The listing builds one solid part. Answer for the finished solid, in the listing's coordinates (mm). Face numbers are marked on the shaded views. A direction names the side the tool comes from. Round coordinates to 2 decimals unless told otherwise and drop trailing zeros. Write each loop counter-clockwise with the first axis right and the second up, starting at its lowest first coordinate (ties: lowest second). Pieces come first, ordered by that corner, then holes.
(1) A cutting plane is placed at A-A, the plane z = 0. Give the vertices of the cut face in (x, y) (3 decimals).
(2) A cutting plane is placed at D-D, the plane x = 34.5. Give the vertices of the cut face in (y, z) (3 decimals), and give its area (3 significant figures).
(3) Each of these flat-tipped pins is pushed along its axis until it touches: pin 1 Ø3 at (x, z) = (59.5, -6) entering from +Y; pin 2 Ø3 at (x, y) = (44, -3.5) entering from +Z; pin 3 Ø8 at (x, z) = (63, -6) entering from -Y; pin 4 Ø10 at (x, y) = (79, -0.5) entering from -Z (3 decimals). Where does it stop, or does it pass through?
(4) For the marked faces 1 and 2, determine the directions among +Z, -Z, +X, -X, +Y, -Y from which every point of the face is accessible in a straight line to the end or side of a thin tool.
(5) Find the intervals of material crossed by probe 1 along X at (y, z) = (3, 5.5); probe 2 along Z at (x, y) = (57, 1.75); probe 3 along Z at (x, y) = (98, -8), in increasing order.
(6) A cutting plane is placed at C-C, the plane x = 103.5. Give the vertices of the cut face in (y, z), and give its area (3 significant figures).
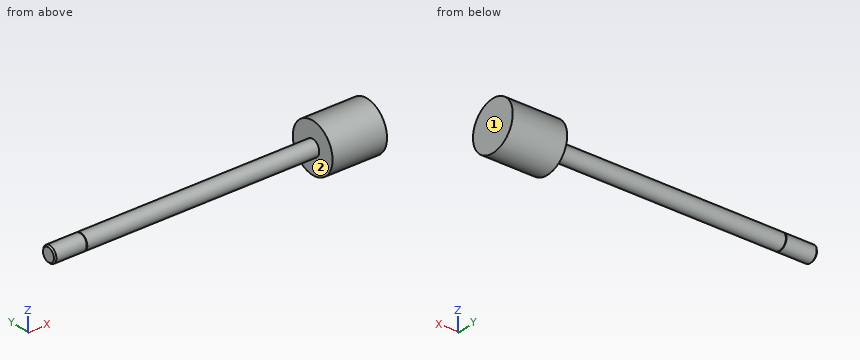
from build123d import *

# Parameters (mm, degrees)
SKETCH3_W = 0.254
SKETCH3_H = 0.508


with BuildPart() as part:
    # Sketch1 → Revolve1 (revolve)
    with BuildSketch(Plane.XY):
        Polygon((0, 0), (0, 3.175), (91.2876, 3.175), (91.2876, 9.62025), (112.7252, 9.62025), (112.7252, 0), align=None)
    revolve(axis=Axis((112.7252, 0, 0), (-1, 0, 0)))

    # Sketch2 → Revolve2 (revolve)
    with BuildSketch(Plane.XY):
        Polygon((-12.7, 0), (-12.7, 2.63398), (-12.15898, 3.175), (0, 3.175), (0, 0), align=None)
    revolve(axis=Axis((0, 0, 0), (-1, 0, 0)))

    # Sketch3 → Cut-Revolve1 (revolve, cut)
    with BuildSketch(Plane.XY):
        with Locations((-0.127, 3.175)):
            Rectangle(SKETCH3_W, SKETCH3_H)
    revolve(axis=Axis((0, 0, 0), (-1, 0, 0)), mode=Mode.SUBTRACT)


solid = part.part
Solutions:
1. outline: (-12.7, -2.634) - (-12.159, -3.175) - (-0.254, -3.175) - (-0.254, -2.921) - (0, -2.921) - (0, -3.175) - (91.288, -3.175) - (91.288, -9.62) - (112.725, -9.62) - (112.725, 9.62) - (91.288, 9.62) - (91.288, 3.175) - (0, 3.175) - (0, 2.921) - (-0.254, 2.921) - (-0.254, 3.175) - (-12.159, 3.175) - (-12.7, 2.634) - close
2. outline: circle Ø6.35 at (0, 0)
2. area: 31.7 mm2
3. pin 1: passes through
3. pin 2: stops at z = 2.47
3. pin 3: stops at y = -2.47
3. pin 4: stops at z = -3.175
4. face 1: +Z, -Z, +X, +Y, -Y
4. face 2: -X
5. probe 1: x = 91.29 to 112.73
5. probe 2: z = -2.65 to 2.65
5. probe 3: z = -5.34 to 5.34
6. outline: circle Ø19.24 at (0, 0)
6. area: 291 mm2
